Autodesk Inventor part; units mm, degrees
ref_plane "YZ Plane" through (0, 0, 0) normal (1, 0, 0) x (0, 1, 0)
ref_plane "XZ Plane" through (0, 0, 0) normal (0, 1, 0) x (-1, 0, 0)
ref_plane "XY Plane" through (0, 0, 0) normal (0, 0, 1) x (1, 0, 0)
sketch "スケッチ2" plane through (-42.95, -21, 0) normal (0, -1, 0) x (1, 0, 0)
  line L0 (0, 0) -> (25.9, 5) construction
  line L1 (0, 5) -> (25.9, 5)
  line L2 (12.95, 5) -> (12.95, 0) construction
  line L3 (0, 0) -> (25.9, 0)
  line L4 (0, 0) -> (0, 5)
  line L5 (0, 2.5) -> (25.9, 2.5) construction
  line L6 (25.9, 0) -> (25.9, 5)
  point P0 (42.95, 0)
  point P1 (2.95, 2.5)
  point P2 (22.95, 2.5)
  dimension "d176" = 20
sketch "スケッチ1" plane through (0, 0, 0) normal (0, 0, 1) x (1, 0, 0)
  line L0 (-72.5, 26) -> (-45, 26) construction
  line L1 (72.5, 26) -> (72.5, 13) construction
  line L2 (-72.5, -26) -> (-72.5, 13)
  line L3 (-72.5, 26) -> (72.5, -26) construction
  line L4 (72.5, 26) -> (-72.5, -26) construction
  line L5 (2.5, 26) -> (2.5, 13)
  line L6 (2.5, 13) -> (4.6, 13) construction
  line L7 (2.5, 26) -> (72.5, 26) construction
  line L8 (72.5, 13) -> (72.5, -26)
  line L9 (70, 13) -> (70, -25.5) construction
  circle A0 centre (67.5, 8) radius 1.55
  line L10 (-31.25, 26) -> (-31.25, 31)
  line L11 (-31.25, 31) -> (-11.25, 31)
  line L12 (-11.25, 31) -> (-11.25, 26)
  line L13 (-31.25, 26) -> (-11.25, 26) construction
  line L14 (-11.25, 26) -> (-9.15, 26) construction
  arc A1 (-33.35, 26) -> (-31.25, 26) centre (-32.3, 26) ccw
  arc A2 (-11.25, 26) -> (-9.15, 26) centre (-10.2, 26) ccw
  line L15 (-33.35, 26) -> (-31.25, 26) construction
  line L16 (-9.15, 26) -> (2.5, 26)
  line L17 (-45.05, -21) -> (-42.95, -21) construction
  arc A3 (-42.95, -21) -> (-45.05, -21) centre (-44, -21) ccw
  arc A4 (-14.95, -21) -> (-17.05, -21) centre (-16, -21) ccw
  line L18 (-42.95, -21) -> (-17.05, -21)
  line L19 (-17.05, -21) -> (-14.95, -21) construction
  line L20 (15, -21) -> (45, -21) construction
  line L21 (45, -21) -> (45, -23.5) construction
  line L22 (45, -23.5) -> (15, -23.5) construction
  line L23 (15, -23.5) -> (15, -21) construction
  line L24 (15, -21) -> (45, -23.5) construction
  line L25 (45, -21) -> (15, -23.5) construction
  line L26 (14.95, -20.95) -> (45.05, -20.95)
  line L27 (45.05, -20.95) -> (45.05, -23.55)
  line L28 (45.05, -23.55) -> (14.95, -23.55)
  line L29 (14.95, -23.55) -> (14.95, -20.95)
  line L30 (14.95, -20.95) -> (45.05, -23.55) construction
  line L31 (45.05, -20.95) -> (14.95, -23.55) construction
  line L32 (-45, -21) -> (-45, -26) construction
  line L33 (-15, -21) -> (-15, -26) construction
  line L34 (72.5, -6.5) -> (-72.5, -6.5) construction
  line L35 (70, 1) -> (67.5, 1) construction
  line L36 (67.5, 1) -> (67.5, -14) construction
  line L37 (67.5, -14) -> (70, -14) construction
  line L38 (70, -14) -> (70, 1) construction
  line L39 (70, 1) -> (67.5, -14) construction
  line L40 (67.5, 1) -> (70, -14) construction
  line L41 (67.45, 1.05) -> (70.05, 1.05)
  line L42 (70.05, 1.05) -> (70.05, -1.05) construction
  line L43 (70.05, -14.05) -> (67.45, -14.05)
  line L44 (67.45, -14.05) -> (67.45, -11.95) construction
  line L45 (67.45, 1.05) -> (70.05, -14.05) construction
  line L46 (70.05, 1.05) -> (67.45, -14.05) construction
  arc A5 (67.45, 1.05) -> (67.45, -1.05) centre (67.45, 0) ccw
  arc A6 (70.05, -1.05) -> (70.05, 1.05) centre (70.05, 0) ccw
  arc A7 (67.45, -11.95) -> (67.45, -14.05) centre (67.45, -13) ccw
  arc A8 (70.05, -14.05) -> (70.05, -11.95) centre (70.05, -13) ccw
  line L47 (67.45, -1.05) -> (67.45, 1.05) construction
  line L48 (67.45, -11.95) -> (67.45, -1.05)
  line L49 (70.05, -11.95) -> (70.05, -14.05) construction
  line L50 (70.05, -1.05) -> (70.05, -11.95)
  circle A9 centre (67.5, -21) radius 1.55
  line L51 (-72.5, -26) -> (-62.5, -26) construction
  line L52 (-15, -26) -> (72.5, -26)
  line L53 (-45, -26) -> (-15, -26) construction
  line L54 (-70, 26.5) -> (-70, -26) construction
  line L55 (-65, 26) -> (-65, -26) construction
  arc A10 (2.5, 13) -> (4.6, 13) centre (3.55, 13) ccw
  line L56 (4.6, 13) -> (72.5, 13)
  circle A11 centre (67.5, 8) radius 3
  circle A12 centre (67.5, -21) radius 3
  line L57 (2.5, 8) -> (2.5, -18)
  line L58 (2.5, -18) -> (52.329, -18)
  line L59 (52.329, -18) -> (6.2717, 8)
  line L60 (16.4427, 8) -> (62.5, 8)
  line L61 (62.5, 8) -> (62.5, -18)
  line L62 (62.5, -18) -> (16.4427, 8)
  line L63 (-62.5, -18) -> (-6.7423, -18)
  line L64 (-6.7423, -18) -> (-42.3875, 8)
  line L65 (-2.5, 21) -> (-2.5, -14.9056)
  line L66 (-2.5, -14.9056) -> (-40, 12.4473)
  line L67 (2.5, 13) -> (2.5, -26) construction
  line L68 (6.2717, 8) -> (2.5, 8)
  line L69 (2.5, 13) -> (71.586, -26) construction
  circle A13 centre (-67.5, -28.5) radius 2.1
  circle A14 centre (-67.5, -2) radius 1.45
  circle A15 centre (-67.5, 3) radius 1.45
  circle A16 centre (-67.5, 8) radius 1.45
  line L70 (-67.5, 26) -> (-67.5, -26) construction
  line L71 (-45.05, -21) -> (-45.05, -26)
  line L72 (-14.95, -21) -> (-14.95, -26)
  line L73 (-45, 26) -> (-45, 22)
  line L74 (-45, 13) -> (-72.5, 13)
  line L75 (-62.5, 8) -> (-42.3875, 8)
  line L76 (-40, 21) -> (-40, 12.4473)
  line L77 (-72.5, -26) -> (-72.5, -33.5)
  line L78 (-72.5, -33.5) -> (-62.5, -33.5)
  line L79 (-62.5, -26) -> (-62.5, -33.5)
  line L80 (-62.5, -26) -> (-45, -26)
  line L81 (-45, 26) -> (-33.35, 26)
  line L82 (-45, 22) -> (-45, 13)
  line L83 (-62.5, 8) -> (-62.5, -18)
  line L84 (-2.5, -18) -> (-45, 13) construction
  line L85 (-45.05, 22) -> (-45, 22)
  line L86 (-40, 21) -> (-2.5, 21)
  line L87 (-72.5, 13) -> (-72.5, 26) construction
  arc A17 (14.95, -23.55) -> (17.05, -23.55) centre (16, -23.55) ccw
  line L88 (14.95, -22.25) -> (45.05, -22.25) construction
  line L89 (30, -20.95) -> (30, -23.55) construction
  arc A18 (17.05, -20.95) -> (14.95, -20.95) centre (16, -20.95) ccw
  arc A19 (42.95, -23.55) -> (45.05, -23.55) centre (44, -23.55) ccw
  arc A20 (45.05, -20.95) -> (42.95, -20.95) centre (44, -20.95) ccw
  point P0 (0, 0)
  point P1 (30, -22.25)
  point P2 (68.75, -6.5)
  point P3 (-60, 14.6054)
  point P4 (-46.25, 11.0112)
  point P5 (-54.1904, 10.5)
  point P6 (-45.5266, 10.5)
  point P7 (42.95, -20.95)
  dimension "d0" = 145
  dimension "d1" = 52
  dimension "d2" = 75
  dimension "d3" = 13
  dimension "d4" = 2.5
  dimension "d5" = 3.1
  dimension "d6" = 2.5
  dimension "d7" = 5
  dimension "d12" = 20
  dimension "d14" = 5
  dimension "d15" = 1.05
  dimension "d16" = 1.05
  dimension "d17" = 70
  dimension "d55" = 1.05
  dimension "d56" = 1.05
  dimension "d74" = 39
  dimension "d107" = 30
  dimension "d108" = 2.5
  dimension "d109" = 0.05
  dimension "d110" = 0.05
  dimension "d116" = 30
  dimension "d124" = 15
  dimension "d125" = 0.05
  dimension "d126" = 0.05
  dimension "d127" = 1.05
  dimension "d128" = 1.05
  dimension "d129" = 1.05
  dimension "d130" = 1.05
  dimension "d132" = 30
  dimension "d134" = 5
  dimension "d135" = 2.5
  dimension "d146" = 5
  dimension "d147" = 20
  dimension "d152" = 1.05
  dimension "d169" = 6
  dimension "d186" = 5
  dimension "d187" = 5
  dimension "d190" = 8
  dimension "d192" = 5
  dimension "d193" = 5
  dimension "d196" = 2.5
  dimension "d200" = 4.2
  dimension "d205" = 2.5
  dimension "d206" = 2.9
  dimension "d207" = 2.9
  dimension "d208" = 2.9
  dimension "d209" = 2.5
  dimension "d211" = 5
  dimension "d212" = 5
  dimension "d213" = 0.05
  dimension "d214" = 0.05
  dimension "d215" = 2.5
  dimension "d216" = 5
  dimension "d217" = 2.5
  dimension "d220" = 18
  dimension "d222" = 13
  dimension "d225" = 13.75
  dimension "d226" = 27.5
  dimension "d227" = 5
  dimension "d228" = 5
  dimension "d233" = 7.5
  dimension "d234" = 2.5
  dimension "d235" = 2.5
  dimension "d236" = 5
extrude "押し出し1" add sketch "スケッチ1" along normal blind 5 contours L2 L74 L82 L73 L81 A1 L10 L11 L12 A2 L16 L5 A10 L56 L8 L52 L72 A4 L18 A3 L71 L80 L79 L78 L77
extrude "押し出し2" add sketch "スケッチ1" along normal blind 2 contours A11 | A12
hole "穴1" at (-40, -21, 2.5) at (-20, -21, 2.5) direction (0, 1, 0) diameter 2.459 depth 5
chamfer "面取り1" distance 2.5 angle 45 5 edges at (72.5, -26, 2.5) (72.5, 13, 2.5) (-72.5, -33.5, 2.5) (-72.5, 13, 2.5) (-62.5, -33.5, 2.5)
fillet "フィレット2" radius 1 11 edges at (-6.7423, -18, 2.5) (-2.5, -14.9056, 2.5) (2.5, -18, 2.5) (2.5, 8, 2.5) (6.2717, 8, 2.5) (16.4427, 8, 2.5) (62.5, 8, 2.5) (62.5, -18, 2.5) (52.329, -18, 2.5) (-45, 13, 2.5) (-62.5, -26, 2.5)
extrude "押し出し4" add sketch "スケッチ1" along normal blind 0.5 contours L68 L59 L58 L57 | L60 L61 L62 | L83 L75 L64 L63 | L65 L66 L76 L86
sketch "スケッチ9" plane through (-45, 26, 0) normal (0, 1, 0) x (1, 0, 0)
  line L0 (33.75, 0) -> (33.75, -5)
  line L1 (13.75, 0) -> (13.75, -5)
  line L2 (33.75, 0) -> (13.75, 0)
  line L3 (47.5, 0) -> (35.85, 0)
  point P0 (45, 0)
  point P1 (8.75, -2.5)
  point P2 (38.75, -2.5)
  dimension "d237" = 20
  dimension "d238" = 30
  dimension "d239" = 5
  dimension "d240" = 2.5
  dimension "d241" = 2.5
hole "穴6" at (-36.25, 26, 2.5) at (-6.25, 26, 2.5) direction (0, -1, 0) diameter 2.459 depth 5
equation "\"d16\" = d15"
equation "\"d55\" = d54"
equation "\"d56\" = d55"
equation "\"d53\" = d15"
equation "\"d54\" = d53"
properties part number "Cockpit_lower_side_frame" material "アセタール樹脂、黒"
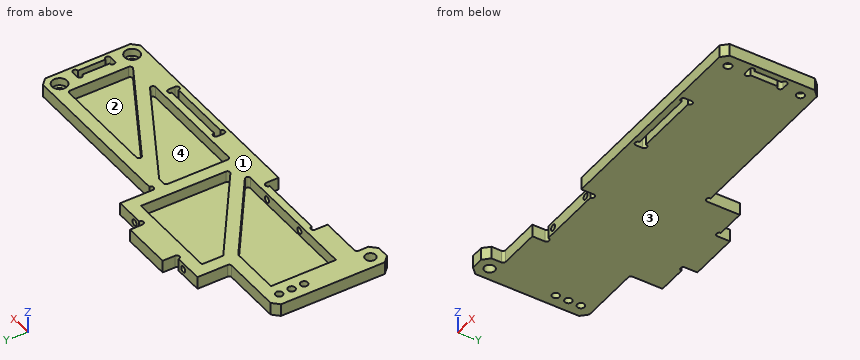
Work out the finished part from the listing and answer in its coordinate system (mm). Face numbers are marked on the shaded views. A direction names the side the tool comes from. Coordinates: 2 decimals unless noted, no trailing zeros. Loops run counter-clockwise (first coordinate to the right, second up) from the corner with the lowest first, then second, coordinate; pieces in that order, holes last. Notation, with made-up numbers: M 16.5,-30.5 L 38.5,-30.5 A20 ccw 38.5,-22.5 Z; hole C 58.25,23 d5. An arc over 180 degrees is marked long. Use CSV: the item, a comma, the result in double quotes. Start each with the question number.
(1) Find section A-A, the plane y = -10.5. Give the vertices of the cut face in (x, z).
(2) Given pin 1 Ø21 at (x, y) = (-27.5, -6.5) entering from +Z; pin 2 Ø1.5 at (x, z) = (26.5, 2.5) entering from +Y; pin 3 Ø3 at (x, z) = (4.5, 3) entering from -Y; pin 4 Ø2.5 at (y, z) = (28, 1.5) entering from +X, each flat-ended and moving along its own axis, determine where each tip first touches the part or whether it passes through.
(3) For the marked faces 3 and 4, determine the directions among +Z, -Z, +X, -X, +Y, -Y from which every point of the face is accessible in a straight line to the end or side of a thin tool.
(4) For a pull along Y with two mould halves and no side action, classify the marked faces 1 and 2 as +Y half, -Y half, draft (parallel to the pull), parting line (faces both ways), or undercut.
(5) Consider line 1 (Y direction, x = 67.5, z = 0.5); line 2 (Y direction, x = -67.5, z = 2.9); line 3 (Y direction, x = -58, z = 3.85). Determine where each line is inside the solid, lowest interval first.
(6) Find section B-B, the plane x = -59. Give the vertices of the cut face in (y, z), then the cut area to 3 significant figures.
Recorded:
1,outline,"M -72.5,0 L 67.45,0 L 67.45,5 L 62.5,5 L 62.5,0.5 L 49.21,0.5 L 49.21,5 L 39.04,5 L 39.04,0.5 L 2.5,0.5 L 2.5,5 L -2.5,5 L -2.5,0.5 L -8.54,0.5 L -8.54,5 L -17.02,5 L -17.02,0.5 L -62.5,0.5 L -62.5,5 L -72.5,5 Z; M 70.05,0 L 72.5,0 L 72.5,5 L 70.05,5 Z"
2,pin 1,"stops at z = 5"
2,pin 2,"stops at y = 13"
2,pin 3,"stops at y = -26"
2,pin 4,"stops at x = -11.25"
3,face 3,"-Z, +X, -X, +Y, -Y"
3,face 4,"+Z"
4,face 1,"draft"
4,face 2,"undercut"
5,line 1,"y = -26 to -22.55, -19.45 to -14.05, 1.05 to 6.45, 9.55 to 13"
5,line 2,"y = -33.5 to -30.6, -26.4 to -3.45, -0.55 to 1.55, 4.45 to 6.55, 9.45 to 13"
5,line 3,"y = -26 to -18, 8 to 13"
6,outline,"M -26,0 L 13,0 L 13,5 L 8,5 L 8,0.5 L -18,0.5 L -18,5 L -26,5 Z"
6,area,"78.0 mm^2"
